```python
from build123d import *

# Parameters (mm, degrees)
SKETCH1_R           = 0.5
SKETCH1_R_2         = 1.1
BOSS_EXTRUDE1_DEPTH = 1.3
SKETCH3_R           = 2.15
CUT_EXTRUDE1_DEPTH  = 1
SKETCH4_R           = 3.4
BOSS_EXTRUDE3_DEPTH = 2.3
SKETCH5_R           = 2.35
CUT_EXTRUDE2_DEPTH  = 1.9
CUT_EXTRUDE3_REACH  = 15.77
SKETCH6_R           = 1.1


with BuildPart() as part:
    # Sketch1 → Boss-Extrude1 (new body)
    with BuildSketch(Plane(origin=(0, 0, 0), x_dir=(1, 0, 0), z_dir=(0, 1, 0))):
        with BuildLine():
            Line((3.766745444, 8.319988196), (-8.208470762, 7.669550455))
            ThreePointArc((-8.208470762, 7.669550455), (-10.1, 5.672494098), (-8.208470762, 3.675437741))
            Line((-8.208470762, 3.675437741), (3.766745444, 3.025))
            ThreePointArc((3.766745444, 3.025), (9.3, 5.672494098), (3.766745444, 8.319988196))
        make_face()
        with Locations(Location((-8.7, 5.672494098, 0), (0, 0, 270))):
            Circle(SKETCH1_R, mode=Mode.SUBTRACT)
        with Locations(Location((1.3, 5.672494098, 0), (0, 0, 270))):
            Circle(SKETCH1_R, mode=Mode.SUBTRACT)
        with Locations(Location((-0.7, 5.672494098, 0), (0, 0, 270))):
            Circle(SKETCH1_R, mode=Mode.SUBTRACT)
        with Locations(Location((-2.7, 5.672494098, 0), (0, 0, 270))):
            Circle(SKETCH1_R, mode=Mode.SUBTRACT)
        with Locations(Location((-4.7, 5.672494098, 0), (0, 0, 270))):
            Circle(SKETCH1_R, mode=Mode.SUBTRACT)
        with Locations(Location((-6.7, 5.672494098, 0), (0, 0, 270))):
            Circle(SKETCH1_R, mode=Mode.SUBTRACT)
        with Locations(Location((5.9, 5.672494098, 0), (0, 0, 270))):
            Circle(SKETCH1_R_2, mode=Mode.SUBTRACT)
    extrude(amount=-BOSS_EXTRUDE1_DEPTH)

    # Sketch3 → Cut-Extrude1 (cut)
    with BuildSketch(Plane(origin=(0, 0, 0), x_dir=(1, 0, 0), z_dir=(0, 1, 0))):
        with Locations(Location((5.9, 5.672494098, 0), (0, 0, 270))):
            Circle(SKETCH3_R)
    extrude(amount=-CUT_EXTRUDE1_DEPTH, mode=Mode.SUBTRACT)

    # Sketch4 → Boss-Extrude3 (add)
    with BuildSketch(Plane.XZ.offset(1.3)):
        with Locations(Location((5.9, -5.672494098, 0), (0, 0, 90))):
            Circle(SKETCH4_R)
    extrude(amount=BOSS_EXTRUDE3_DEPTH)

    # Sketch5 → Cut-Extrude2 (cut)
    with BuildSketch(Plane.XZ.offset(3.6)):
        with Locations(Location((5.9, -5.672494098, 0), (0, 0, 270))):
            Circle(SKETCH5_R)
    extrude(amount=-CUT_EXTRUDE2_DEPTH, mode=Mode.SUBTRACT)

    # Sketch6 → Cut-Extrude3 (cut, up to next)
    with BuildSketch(Plane(origin=(0, -1.3, 0), x_dir=(1, 0, 0), z_dir=(0, 1, 0)), mode=Mode.PRIVATE) as cut_extrude3_sk1:
        with Locations(Location((5.9, 5.672494098, 0), (0, 0, 270))):
            Circle(SKETCH6_R)
    cut_extrude3_tool1 = extrude(cut_extrude3_sk1.sketch, amount=-CUT_EXTRUDE3_REACH, mode=Mode.PRIVATE) & part.part
    add(cut_extrude3_tool1.solids().sort_by_distance((5.9, -1.3, -5.672494))[0], mode=Mode.SUBTRACT)


solid = part.part
```
Model file for the job. Use its own axes, mm. A direction names the side the tool comes from. Round coordinates to 2 decimals unless told otherwise and drop trailing zeros. Write each loop counter-clockwise with the first axis right and the second up, starting at its lowest first coordinate (ties: lowest second). Pieces come first, ordered by that corner, then holes. Notation, with made-up numbers: (54.25, 88.25) - (76.25, 88.25) arc R20 cw to (76.25, 118.25) - close; hole circle Ø5 at (84, 61.5). An arc over 180 degrees is marked (long way). Use CSV: the item, a comma, the result in double quotes. Start each with the question number.
Item 1: Tool access for faces 5 (the face through (5.077, -0.493, -3.686)), 6 (the face through (-8.678, -0.641, -6.172)), 7 (the face through (5, -1.7, -7)): list every direction of +Z, -Z, +X, -X, +Y, -Y with a clear straight run to the whole face (end or side of a thin tool).
Item 2: Pin check, flat tips, straight feed: P1, Ø1.5, axis at y = -0.5, z = -7, coming from the -X side; P2, Ø1.3, axis at x = 5.9, z = -5.67, coming from the +Y side; P3, Ø1, axis at x = 0.5, y = -1.5, coming from the -Z side; P4, Ø1.3, axis at x = 5, z = -6.5, coming from the +Y side. Stop position of each tip, or through.
Item 3: Band-saw the part on A-A (y = -0.5). State how many separate pieces and enclosed holes the cut face has, and give its area (3 significant figures).
Item 4: Band-saw the part on B-B (x = 5.9). Write the cut outline in (y, z), and give its area (3 significant figures).
Item 5: Drill centre lines: L1, parallel to Y at x = -1.5, z = -7; L2, parallel to X at y = -3.2, z = -6.5; L3, parallel to X at y = -0.65, z = -7.5. Where is each one in solid material? Low to high. Write a range as [from, to].
Item 6: Two-plate mould, pull along X, no slides. Class faces 1 (the face through (-2.305, -0.641, -3.355)), 2 (the face through (6, -1, -7)), 3 (the face through (-0.678, -0.641, -6.172)), 4 (the face through (5, -3.6, -3)): released by +X, released by -X, zero draft, split by the parting line, or undercut.
Item 7: Band-saw the part on C-C (z = -4.75). Write the cut outline in (x, y), and give its area (3 significant figures).
Item 8: Band-saw the part on D-D (y = -2.65). Write the cut outline in (x, z), and give its area (3 significant figures).
Checked values:
1,face 5,"+Y"
1,face 6,"+Y, -Y"
1,face 7,"-Y"
2,P1,"stops at x = -10.01"
2,P2,"passes through"
2,P3,"stops at z = -8.17"
2,P4,"stops at y = -1"
3,separate pieces,"1"
3,enclosed holes,"7"
3,area,"73.9 mm²"
4,outline,"(-3.6, -9.07) - (0, -9.07) - (0, -7.82) - (-1, -7.82) - (-1, -6.77) - (-1.7, -6.77) - (-1.7, -8.02) - (-3.6, -8.02) - close; (-3.6, -3.32) - (-1.7, -3.32) - (-1.7, -4.57) - (-1, -4.57) - (-1, -3.52) - (0, -3.52) - (0, -2.27) - (-3.6, -2.27) - close"
4,area,"9.71 mm²"
5,L1,"y = [-1.3, 0]"
5,L2,"x = [2.6, 3.7], [8.1, 9.2]"
5,L3,"x = [-8.91, 4.77], [7.03, 8.77]"
6,face 1,"released by -X"
6,face 2,"undercut"
6,face 3,"undercut"
6,face 4,"zero draft"
7,outline,"(-9.87, -1.3) - (2.63, -1.3) - (2.63, -3.6) - (3.74, -3.6) - (3.74, -1.7) - (5.3, -1.7) - (5.3, -1) - (3.96, -1) - (3.96, 0) - (-9.87, 0) - close; (6.5, -1.7) - (8.06, -1.7) - (8.06, -3.6) - (9.17, -3.6) - (9.17, 0) - (7.84, 0) - (7.84, -1) - (6.5, -1) - close"
7,area,"26.9 mm²"
8,outline,"circle Ø6.8 at (5.9, -5.67); hole circle Ø4.7 at (5.9, -5.67)"
8,area,"19.0 mm²"
